from build123d import *

# Parameters (mm, degrees)
SKETCH_1_R          = 22
EXTRUDE_1_DEPTH     = 20
SKETCH_2_R          = 12.079771489
EXTRUDE_2_DEPTH     = 460
SKETCH_3_R          = 17
EXTRUDE_3_DEPTH     = 20
SKETCH_4_R          = 8
CUT_EXTRUDE_1_DEPTH = 501
SKETCH_5_R          = 13
CUT_EXTRUDE_2_DEPTH = 19


with BuildPart() as part:
    # 草图1 → 凸台-拉伸1 (new body)
    with BuildSketch(Plane(origin=(0, 0, 0), x_dir=(1, 0, 0), z_dir=(0, 1, 0))):
        Circle(SKETCH_1_R)
    extrude(amount=EXTRUDE_1_DEPTH)

    # 草图2 → 凸台-拉伸2 (add)
    with BuildSketch(Plane(origin=(0, 20, 0), x_dir=(1, 0, 0), z_dir=(0, 1, 0))):
        Circle(SKETCH_2_R)
    extrude(amount=EXTRUDE_2_DEPTH)

    # 草图3 → 凸台-拉伸3 (add)
    with BuildSketch(Plane(origin=(0, 480, 0), x_dir=(1, 0, 0), z_dir=(0, 1, 0))):
        Circle(SKETCH_3_R)
    extrude(amount=EXTRUDE_3_DEPTH)

    # 草图4 → 切除-拉伸1 (cut, through all)
    with BuildSketch(Plane.XZ):
        Circle(SKETCH_4_R)
    extrude(amount=-CUT_EXTRUDE_1_DEPTH, mode=Mode.SUBTRACT)

    # 草图5 → 切除-拉伸2 (cut)
    with BuildSketch(Plane(origin=(0, 500, 0), x_dir=(1, 0, 0), z_dir=(0, 1, 0))):
        Circle(SKETCH_5_R)
    extrude(amount=-CUT_EXTRUDE_2_DEPTH, mode=Mode.SUBTRACT)


solid = part.part
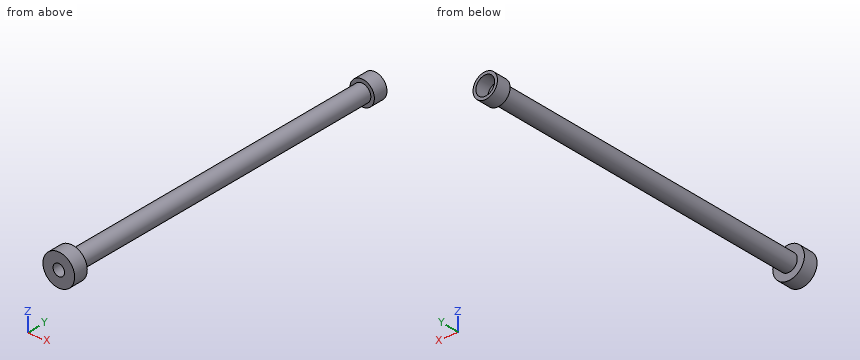
The model under review builds one solid part; all positions refer to its coordinate system, in mm. Coordinates: 2 decimals unless noted, no trailing zeros. Write each loop counter-clockwise with the first axis right and the second up, starting at its lowest first coordinate (ties: lowest second). Pieces come first, ordered by that corner, then holes. Notation, with made-up numbers: (9.5, -17.5) - (31.5, -17.5) arc R21 cw to (31.5, 15.5) - close; hole circle Ø7 at (-5.75, 33). An arc over 180 degrees is marked (long way). Answer as a JSON object with one key per item and string values. Group by question number.
1. Add section B-B (x = 0). Give the boundary of the cut face in (y, z).
2. Add section C-C (y = 389.5). Give the boundary of the cut face in (x, z), plus the area to 3 significant figures.
3. Add section A-A (z = 0). Give the boundary of the cut face in (x, y), plus the area to 3 significant figures.
4. Clearance check with flat-ended pins moving along their axes: pin 1 Ø4 at (x, y) = (10, 274) entering from -Z; pin 2 Ø4 at (x, y) = (-5.5, 87) entering from +Z; pin 3 Ø12 at (y, z) = (282, -7) entering from +X. State where each tip first meets the part, or that it passes through.
5. To check wall thickness, follow probe 1 along Z at (x, y) = (0, 255); probe 2 along X at (y, z) = (486, 0); probe 3 along Y at (x, z) = (0, -16.5). State the ranges of each line that lie inside material, in increasing order.
Findings:
{
 "1": {"outline": "(0, -22) - (20, -22) - (20, -12.08) - (480, -12.08) - (480, -17) - (500, -17) - (500, -13) - (481, -13) - (481, -8) - (0, -8) - close; (0, 8) - (481, 8) - (481, 13) - (500, 13) - (500, 17) - (480, 17) - (480, 12.08) - (20, 12.08) - (20, 22) - (0, 22) - close"},
 "2": {"outline": "circle Ø24.16 at (0, 0); hole circle Ø16 at (0, 0)", "area": "257 mm²"},
 "3": {"outline": "(-22, 0) - (-8, 0) - (-8, 481) - (-13, 481) - (-13, 500) - (-17, 500) - (-17, 480) - (-12.08, 480) - (-12.08, 20) - (-22, 20) - close; (8, 0) - (22, 0) - (22, 20) - (12.08, 20) - (12.08, 480) - (17, 480) - (17, 500) - (13, 500) - (13, 481) - (8, 481) - close", "area": "4,480 mm²"},
 "4": {"pin 1": "z = -9.05", "pin 2": "z = 11.56", "pin 3": "x = 12.04"},
 "5": {"probe 1": "-12.08 to -8, 8 to 12.08", "probe 2": "-17 to -13, 13 to 17", "probe 3": "0 to 20, 480 to 500"}
}
